Autodesk Inventor part; units mm, degrees
ref_plane "YZ Plane" through (0, 0, 0) normal (1, 0, 0) x (0, 1, 0)
ref_plane "XZ Plane" through (0, 0, 0) normal (0, 1, 0) x (-1, 0, 0)
ref_plane "XY Plane" through (0, 0, 0) normal (0, 0, 1) x (1, 0, 0)
sketch "Sketch1" plane through (0, 0, 0) normal (0, 0, 1) x (1, 0, 0)
  line L0 (-17.78, 0) -> (17.78, 0)
  line L1 (0, -17.78) -> (0, 17.78)
  line L2 (-12.7, 12.7) -> (12.7, 12.7)
  line L3 (12.7, 12.7) -> (12.7, -12.7)
  line L4 (12.7, -12.7) -> (-12.7, -12.7)
  line L5 (-12.7, -12.7) -> (-12.7, 12.7)
  line L6 (9.525, 9.525) -> (-9.525, 9.525)
  line L7 (-9.525, 9.525) -> (-9.525, -9.525)
  line L8 (-9.525, -9.525) -> (9.525, -9.525)
  line L9 (9.525, -9.525) -> (9.525, 9.525)
  point P0 (0, 0)
  point P1 (-12.7, 0)
  point P2 (0, 12.7)
  dimension "d0" = 25.4
  dimension "d1" = 3.175
extrude "Extrusion1" add sketch "Sketch1" along normal mid plane 177.8 contours L5 L2 L1 L6 L7 L0 | L0 L7 L8 L1 L4 L5 | L1 L8 L9 L0 L3 L4 | L2 L3 L0 L9 L6 L1
sketch "Sketch3" plane through (-12.7, 12.7, 88.9) normal (0, 1, 0) x (1, 0, 0)
  line L0 (0, 0) -> (25.4, 0)
  line L1 (25.4, 0) -> (25.4, 177.8)
  line L2 (0, 177.8) -> (0, 0)
  line L3 (0, 88.9) -> (25.4, 88.9) construction
  line L4 (0, 0) -> (25.4, 14.6647)
  line L5 (0, 0) -> (25.4, 0)
  line L6 (25.4, 0) -> (25.4, 14.6647)
  line L7 (0, 177.8) -> (25.4, 163.1353)
  line L8 (0, 177.8) -> (25.4, 177.8)
  line L9 (25.4, 177.8) -> (25.4, 163.1353)
  point P0 (12.7, 88.9)
  dimension "d7" = 30
extrude "Extrusion3" cut sketch "Sketch3" against normal through all contours L4 L1 L0 | L8 L1 L7
properties part number "tubing_template_0.125" material "Aluminum-6061"
Design review of the part built by this model. Coordinates are the model's own, in mm. A direction names the side the tool comes from. Round coordinates to 2 decimals unless told otherwise and drop trailing zeros. Write each loop counter-clockwise with the first axis right and the second up, starting at its lowest first coordinate (ties: lowest second). Pieces come first, ordered by that corner, then holes. Notation, with made-up numbers: (-23, 16.25) -> (-9, 16.25) arc R19 cw to (-9, 36.25) -> close; hole circle Ø11 at (-24.75, 35). An arc over 180 degrees is marked (long way). Answer in a Markdown table with one row per item.
Q1. Take a section at B-B, the plane z = -12. State the section outline as (x, y) points (3 decimals), then the cut area to 3 significant figures.
The answers:
| item | result |
|---|---|
| outline | (-12.7, -12.7) -> (12.7, -12.7) -> (12.7, 12.7) -> (-12.7, 12.7) -> close; hole (-9.525, -9.525) -> (9.525, -9.525) -> (9.525, 9.525) -> (-9.525, 9.525) -> close |
| area | 282 mm² |
Q2. Clearance check with a flat-ended pin moving along its axis: pin 1 Ø1.5 at (x, y) = (9.5, -9.5) entering from -Z. State where the tip first meets the part, or that it passes through.
The answers:
| item | result |
|---|---|
| pin 1 | z = -76.52 |
Q3. Draft analysis for pull direction Y (two halves, no side actions). For faces 1 (the face through (0, 9.525, -1)), 2 (the face through (-0.18, -11.11, -81.67)), 3 (the face through (0, -12.7, -1)), 4 (the face through (0, 12.7, -1)), state which applies: +Y half, -Y half, draft (parallel to the pull), parting line (faces both ways), or undercut.
The answers:
| item | result |
|---|---|
| face 1 | undercut |
| face 2 | draft |
| face 3 | -Y half |
| face 4 | +Y half |
Q4. For faces 5 (the face through (9.525, 0, -1)), 6 (the face through (12.7, 0, -1)), list the 3-axis set-ups (+Z, -Z, +X, -X, +Y, -Y) from which the entire face can be reached by the end or side of a thin tool; tool diameter is ignored.
The answers:
| item | result |
|---|---|
| face 5 | +Z, -Z |
| face 6 | +Z, -Z, +X, +Y, -Y |
Q5. Take a section at A-A, the plane y = -5.75. State the section outline as (x, z) points (3 decimals).
The answers:
| item | result |
|---|---|
| outline | (-12.7, -88.9) -> (-9.525, -87.067) -> (-9.525, 87.067) -> (-12.7, 88.9) -> close; (9.525, -76.068) -> (12.7, -74.235) -> (12.7, 74.235) -> (9.525, 76.068) -> close |
Q6. To check wall thickness, follow L1, parallel to Y at x = 7.5, z = -54 (3 decimals); L2, parallel to Z at x = -9.5, y = 10.75. State the ranges of each line that lie inside material, in increasing order. Write a range as [from, to].
The answers:
| item | result |
|---|---|
| L1 | [-12.7, -9.525], [9.525, 12.7] |
| L2 | [-87.05, 87.05] |
Q7. Take a section at C-C, the plane x = 6.75. State the section outline as (y, z) points (3 decimals), then the cut area to 3 significant figures.
The answers:
| item | result |
|---|---|
| outline | (-12.7, -77.671) -> (-9.525, -77.671) -> (-9.525, 77.671) -> (-12.7, 77.671) -> close; (9.525, -77.671) -> (12.7, -77.671) -> (12.7, 77.671) -> (9.525, 77.671) -> close |
| area | 986 mm² |
